Check sheet for the modelled part. Datum: model origin and axes. Units: mm. Face numbers are marked on the shaded views. A direction names the side the tool comes from. Give positions to 0.01 mm unless a question says otherwise; leave off trailing zeros. Order: outer loops, then holes, each group sorted by start corner. A loop starts at its lowest first (then second) coordinate and runs counter-clockwise, first axis right, second up. Notation, with made-up numbers: (-21, 17.25) - (0, 17.25) arc R23 ccw to (0, 37.25) - close; hole circle Ø4 at (17.25, 77). An arc over 180 degrees is marked (long way). Answer in a Markdown table with one row per item.
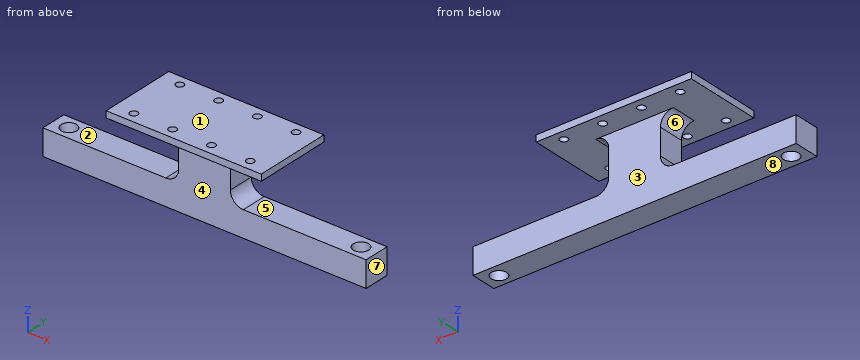
from build123d import *

# Parameters (mm, degrees)
F0_W      = 120
F0_H      = 60
F1_DEPTH  = 5
F2_W      = 40
F2_H      = 20
F3_DEPTH  = 40
F4_W      = 250
F4_H      = 20
F5_DEPTH  = 20
F6_R      = 10
F7_R      = 6
F8_DEPTH  = 65.001
F9_R      = 3
F10_DEPTH = 65.001


with BuildPart() as f1:
    # F0 (on Top) → F1 (new body)
    with BuildSketch(Plane.XY):
        Rectangle(F0_W, F0_H)
    extrude(amount=F1_DEPTH)

    # F2 (on face) → F3 (join)
    with BuildSketch(Plane(origin=(0, 0, 0), x_dir=(1, 0, 0), z_dir=(0, 0, -1))):
        Rectangle(F2_W, F2_H)
    extrude(amount=F3_DEPTH)

    # F4 (on face) → F5 (join)
    with BuildSketch(Plane(origin=(0, 0, -40), x_dir=(1, 0, 0), z_dir=(0, 0, -1))):
        Rectangle(F4_W, F4_H)
    extrude(amount=F5_DEPTH)

    # F6
    f6_edges = [f1.edges().sort_by_distance(p)[0] for p in [
        (-20, 0, -40),
        (20, 0, -40),
        (20, 0, 0),
        (-20, 0, 0),
    ]]
    fillet(f6_edges, radius=F6_R)

    # F7 (on face) → F8 (cut, through all)
    with BuildSketch(Plane(origin=(0, 0, -60), x_dir=(1, 0, 0), z_dir=(0, 0, -1))):
        with Locations((-113, 0)):
            Circle(F7_R)
        with Locations((113, 0)):
            Circle(F7_R)
    extrude(amount=-F8_DEPTH, mode=Mode.SUBTRACT)

    # F9 (on face) → F10 (cut, through all)
    with BuildSketch(Plane.XY.offset(5)):
        with Locations((-15, 22)):
            Circle(F9_R)
        with Locations((15, 22)):
            Circle(F9_R)
        with Locations((-15, -22)):
            Circle(F9_R)
        with Locations((15, -22)):
            Circle(F9_R)
        with Locations((-45, 22)):
            Circle(F9_R)
        with Locations((-45, -22)):
            Circle(F9_R)
        with Locations((45, 22)):
            Circle(F9_R)
        with Locations((45, -22)):
            Circle(F9_R)
    extrude(amount=-F10_DEPTH, mode=Mode.SUBTRACT)


solid = f1.part
(1) Thickness scan on L1, parallel to Y at x = -15, z = 2.4; L2, parallel to X at y = 0, z = -53.25; L3, parallel to Y at x = 113, z = -44.5. Record the ranges inside material, lowest first.
Geometry says:
| item | result |
|---|---|
| L1 | -30 to -25, -19 to 19, 25 to 30 |
| L2 | -125 to -119, -107 to 107, 119 to 125 |
| L3 | -10 to -6, 6 to 10 |
(2) Cross-section at D-D, the plane y = 2.5. Record the cut outline in (x, z), then the cut area to 3 significant figures.
Geometry says:
| item | result |
|---|---|
| outline | (-125, -60) - (-118.45, -60) - (-118.45, -40) - (-125, -40) - close; (-107.55, -60) - (107.55, -60) - (107.55, -40) - (30, -40) arc R10 cw to (20, -30) - (20, -10) arc R10 cw to (30, 0) - (60, 0) - (60, 5) - (-60, 5) - (-60, 0) - (-30, 0) arc R10 cw to (-20, -10) - (-20, -30) arc R10 cw to (-30, -40) - (-107.55, -40) - close; (118.45, -60) - (125, -60) - (125, -40) - (118.45, -40) - close |
| area | 6,850 mm² |
(3) Gauge pin test, flat ends, axial feed: P1, Ø7, axis at x = -15, y = -22, coming from the +Z side; P2, Ø7, axis at x = -15, y = 22, coming from the -Z side; P3, Ø5.5, axis at x = -45, y = 22, coming from the +Z side; P4, Ø19, axis at x = 113, y = 0, coming from the +Z side. Record the tip position at first contact, or that the pin passes through.
Geometry says:
| item | result |
|---|---|
| P1 | z = 5 |
| P2 | z = 0 |
| P3 | through |
| P4 | z = -40 |
(4) Mould release check, pull along Z, two halves, no side actions. Record for the marked faces 6, 7 and 8: pulls with the +Z half, pulls with the -Z half, needs draft (parallel to the pull), parting line crosses it, or undercut.
Geometry says:
| item | result |
|---|---|
| face 6 | undercut |
| face 7 | needs draft |
| face 8 | pulls with the -Z half |
(5) Cross-section at A-A, the plane x = -45. Record the cut outline in (y, z).
Geometry says:
| item | result |
|---|---|
| outline | (-30, 0) - (-25, 0) - (-25, 5) - (-30, 5) - close; (-19, 0) - (19, 0) - (19, 5) - (-19, 5) - close; (-10, -60) - (10, -60) - (10, -40) - (-10, -40) - close; (25, 0) - (30, 0) - (30, 5) - (25, 5) - close |
(6) Cross-section at B-B, the plane y = 22. Record the cut outline in (x, z).
Geometry says:
| item | result |
|---|---|
| outline | (-60, 0) - (-48, 0) - (-48, 5) - (-60, 5) - close; (-42, 0) - (-18, 0) - (-18, 5) - (-42, 5) - close; (-12, 0) - (12, 0) - (12, 5) - (-12, 5) - close; (18, 0) - (42, 0) - (42, 5) - (18, 5) - close; (48, 0) - (60, 0) - (60, 5) - (48, 5) - close |
(7) Cross-section at C-C, the plane x = 33. Record the cut outline in (y, z), then the cut area to 3 significant figures.
Geometry says:
| item | result |
|---|---|
| outline | (-30, 0) - (30, 0) - (30, 5) - (-30, 5) - close; (-10, -60) - (10, -60) - (10, -40) - (-10, -40) - close |
| area | 700 mm² |
(8) Access from +Z, -Z, +X, -X, +Y, -Y to the whole of each face (thin tool, end or side, straight path). Record for the marked faces 1, 2, 3, 4 and 5.
Geometry says:
| item | result |
|---|---|
| face 1 | +Z, +X, -X, +Y, -Y |
| face 2 | -X, +Y, -Y |
| face 3 | -Z, +X, -X, +Y |
| face 4 | -Z, +X, -X, -Y |
| face 5 | +X, +Y, -Y |
